Here's how the part is built. I have some questions about the finished solid (model axes, mm). Coordinates: 2 decimals unless noted, no trailing zeros. Write each loop counter-clockwise with the first axis right and the second up, starting at its lowest first coordinate (ties: lowest second). Pieces come first, ordered by that corner, then holes.
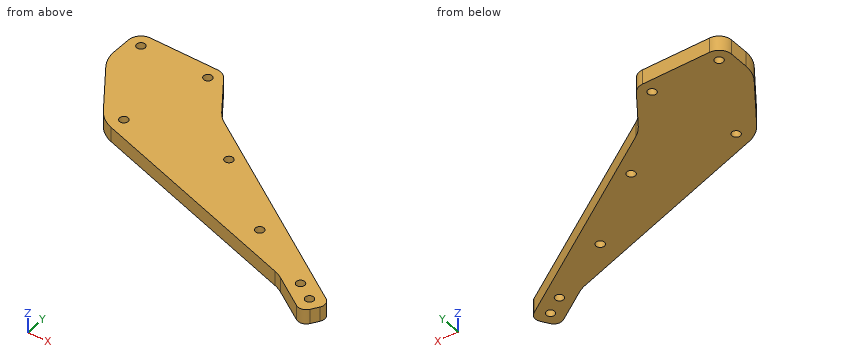
Autodesk Inventor part; units mm, degrees
ref_plane "YZ Plane" through (0, 0, 0) normal (1, 0, 0) x (0, 1, 0)
ref_plane "XZ Plane" through (0, 0, 0) normal (0, 1, 0) x (-1, 0, 0)
ref_plane "XY Plane" through (0, 0, 0) normal (0, 0, 1) x (1, 0, 0)
sketch "Sketch1" plane through (0, 0, 0) normal (0, 0, 1) x (1, 0, 0)
  line L0 (0, 0) -> (22, 0)
  circle A0 centre (3, -3) radius 1
  circle A1 centre (19, -3) radius 1
  circle A2 centre (19, -3) radius 3
  circle A3 centre (3, -3) radius 3
  line L1 (0, -10) -> (27.5638, -10) construction
  line L2 (22, 0) -> (30.0637, -11.5162) construction
  line L3 (22, 0) -> (36.0586, 0) construction
  line L4 (0, -10) -> (0, -3)
  line L5 (28.3404, -11.1091) -> (21.4575, -1.2793)
  line L6 (0, -10) -> (10.7416, -25.3406)
  circle A4 centre (26.0021, -13) radius 1 construction
  line L7 (28.3404, -11.1091) -> (79, -44.0078)
  line L8 (28.3404, -11.1091) -> (26.0021, -13) construction
  line L9 (26.0021, -13) -> (10.7416, -25.3406) construction
  circle A5 centre (13.8594, -22.8194) radius 1
  line L10 (79, -101.0698) -> (79, 42.0759) construction
  line L11 (79, -44.0078) -> (75.7322, -49.0399)
  circle A6 centre (74.8501, -44.8899) radius 1
  line L12 (75.7322, -49.0399) -> (65.6681, -42.5042)
  circle A7 centre (70.6567, -42.1667) radius 1
  line L13 (65.6681, -42.5042) -> (10.7416, -25.3406)
  circle A8 centre (13.8594, -22.8194) radius 3 construction
  circle A9 centre (26.0021, -13) radius 3 construction
  line L14 (67.4577, -36.7773) -> (-2.3075, -14.9769) construction
  line L15 (-2.3075, -14.9769) -> (-9.5668, -6) construction
  line L16 (90.7322, -58.781) -> (24.0944, -15.5059) construction
  line L17 (24.0944, -15.5059) -> (16.5425, -4.7207) construction
  line L18 (47.0108, -30.388) -> (1.9372, -16.3033) construction
  line L19 (1.9372, -16.3033) -> (12.3526, -7.8807) construction
  line L20 (12.3526, -7.8807) -> (47.0108, -30.388) construction
  line L21 (0, -6) -> (22, -6) construction
  line L22 (-9.5668, -6) -> (17.4383, -6) construction
  line L23 (17.4383, -6) -> (22.4483, -13.155) construction
  line L24 (22.4483, -13.155) -> (6.5898, -25.9792) construction
  line L25 (6.5898, -25.9792) -> (-9.5668, -6) construction
  circle A10 centre (54.6727, -33.8896) radius 1
  circle A11 centre (37.1374, -20.399) radius 1
  circle A12 centre (37.1374, -20.399) radius 3 construction
  point P0 (19, 0)
  point P1 (3, 0)
  dimension "d0" = 22
  dimension "d1" = 2
  dimension "d2" = 2
  dimension "d3" = 16
  dimension "d4" = 3
  dimension "d5" = 3
  dimension "d6" = 2
  dimension "d7" = 2
  dimension "d8" = 10
  dimension "d9" = 55
  dimension "d10" = 2
  dimension "d11" = 13
  dimension "d12" = 3
  dimension "d13" = 158
  dimension "d14" = 2
  dimension "d15" = 4
  dimension "d17" = 60
  dimension "d19" = 2
  dimension "d20" = 6
  dimension "d21" = 3
  dimension "d22" = 3
  dimension "d23" = 12
  dimension "d24" = 6
  dimension "d25" = 2
  dimension "d26" = 5
  dimension "d27" = 12
  dimension "d28" = 3
  dimension "d29" = 2
  dimension "d30" = 2
  dimension "d31" = 6
  dimension "d32" = 6
  dimension "d33" = 6
  dimension "d40" = 2
  dimension "d41" = 18
  dimension "d42" = 2
  dimension "d43" = 6
extrude "Extrusion1" add sketch "Sketch1" along normal blind 3.5
fillet "Fillet2" radius 8 4 edges at (10.7416, -25.3406, 1.75) (0, -10, 1.75) (28.3404, -11.1091, 1.75) (65.6681, -42.5042, 1.75)
fillet "Fillet3" radius 2 2 edges at (79, -44.0078, 1.75) (75.7322, -49.0399, 1.75)
equation "\"d24\" = d20"
properties part number "Tibia_V2"
1) I need wall thicknesses on probe 1 along Y at (x, z) = (19, 1.5); probe 2 along Y at (x, z) = (54.5, 0.9); probe 3 along Y at (x, z) = (69, 2.35). Which ranges of each line are inside material? Lowest first, please.
Values follow:
probe 1: y = -27.92 to -4, -2 to 0
probe 2: y = -39.01 to -34.87, -32.9 to -28.1
probe 3: y = -44.67 to -37.51
2) Imagine slicing it at C-C on x = 52. Please give me the cut outline in (y, z), then the cut area to 3 significant figures.
Values follow:
outline: (-38.23, 0) - (-26.47, 0) - (-26.47, 3.5) - (-38.23, 3.5) - close
area: 41.2 mm2
3) Imagine slicing it at B-B on y = -31.5. Please give me the cut outline in (x, z), then the cut area to 3 significant figures.
Values follow:
outline: (30.45, 0) - (59.74, 0) - (59.74, 3.5) - (30.45, 3.5) - close
area: 103 mm2
4) Imagine slicing it at A-A on z = 2.5. Please give me the cut outline in (x, y), then the cut area to 3 significant figures.
Values follow:
outline: (0, -7.48) arc R8 ccw to (1.45, -12.07) - (9.18, -23.11) arc R8 ccw to (13.34, -26.15) - (64.62, -42.18) arc R8 cw to (66.59, -43.1) - (74.05, -47.95) arc R2 ccw to (76.82, -47.36) - (77.91, -45.69) arc R2 ccw to (77.32, -42.92) - (29.64, -11.96) arc R8 cw to (27.45, -9.84) - (21.46, -1.28) arc R3 ccw to (19, 0) - (3, 0) arc R3 ccw to (0, -3) - close; hole circle Ø2 at (3, -3); hole circle Ø2 at (13.86, -22.82); hole circle Ø2 at (19, -3); hole circle Ø2 at (37.14, -20.4); hole circle Ø2 at (54.67, -33.89); hole circle Ø2 at (70.66, -42.17); hole circle Ø2 at (74.85, -44.89)
area: 1,200 mm2
5) Will these pins go through, and if not, where does the flat tip stop? pin 1 (1.6 mm diameter, centred on x = 70.66, y = -42.17, fed in from +Z); pin 2 (2.5 mm diameter, centred on x = 74.85, y = -44.89, fed in from +Z); pin 3 (1 mm diameter, centred on y = -12, z = 3, fed in from +X).
Values follow:
pin 1: passes through
pin 2: stops at z = 3.5
pin 3: stops at x = 30.48
